Here's how the part is built. I have some questions about the finished solid (model axes, mm). Round coordinates to 2 decimals unless told otherwise and drop trailing zeros. Write each loop counter-clockwise with the first axis right and the second up, starting at its lowest first coordinate (ties: lowest second). Pieces come first, ordered by that corner, then holes. Notation, with made-up numbers: (-16.5, 29) - (23.5, 29) arc R18 ccw to (23.5, 34) - close; hole circle Ø9 at (74, 47.5). An arc over 180 degrees is marked (long way). Write item = value, one per line. Start each with the question number.
Item 1: If I drill on line 1 along Z through (x, y) = (110, 16.5); line 2 along Z through (x, y) = (108, 15.5), over which ranges is the centre line in solid material (lowest first)? Write a range as [from, to].
Item 2: For P1, Ø8, axis at x = 94, y = -9, coming from the +Z side; P2, Ø1, axis at x = 118.5, z = -6.5, coming from the +Y side; P3, Ø10, axis at x = 76, y = 11.5, coming from the +Z side, each with a flat end and sliding along its axis, tell me the tip position at first contact or that it passes through.
Item 3: If we section it at A-A (x = 43): Please give me the cut outline in (y, z), and give its area (3 significant figures).
Item 4: If we section it at D-D (x = 110.5): Please give me the cut outline in (y, z).
Item 5: If we section it at C-C (y = 1.5): Please give me the cut outline in (x, z), and give its area (3 significant figures).
Item 6: If we section it at B-B (z = 6): Please give me the cut outline in (x, y).
```python
from build123d import *

# Parameters (mm, degrees)
F0_W     = 20
F0_H     = 30
F1_DEPTH = 17.5
F2_R     = 5


with BuildPart() as f1:
    # F0 (on Front) → F1 (new body, symmetric)
    with BuildSketch(Plane.XZ):
        Rectangle(F0_W, F0_H)
        Polygon((160, -15), (10, 15), (10, -15), align=None)
    extrude(amount=F1_DEPTH, both=True)

    # F2
    f2_edges = [f1.edges().sort_by_distance(p)[0] for p in [
        (-10, 0, 15),
        (-10, -17.5, 0),
        (-10, 17.5, 0),
        (0, -17.5, 15),
        (0, 17.5, 15),
    ]]
    fillet(f2_edges, radius=F2_R)


solid = f1.part
```
Reply:
q1.line_1 = [-15, -5]
q1.line_2 = [-15, -4.6]
q2.P1 = -1
q2.P2 = 17.5
q2.P3 = 2.8
q3.outline = (-17.5, -15) - (17.5, -15) - (17.5, 8.4) - (-17.5, 8.4) - close
q3.area = 819 mm2
q4.outline = (-17.5, -15) - (17.5, -15) - (17.5, -5.1) - (-17.5, -5.1) - close
q5.outline = (-10, -15) - (160, -15) - (10, 15) - (-5, 15) arc R5 ccw to (-10, 10) - close
q5.area = 2,840 mm2
q6.outline = (-10, -12.5) arc R5 ccw to (-5, -17.5) - (55, -17.5) - (55, 17.5) - (-5, 17.5) arc R5 ccw to (-10, 12.5) - close
